CAD build for the part. Positions are in the model's coordinates, mm. Coordinates: 2 decimals unless noted, no trailing zeros. Loops run counter-clockwise (first coordinate to the right, second up) from the corner with the lowest first, then second, coordinate; pieces in that order, holes last. Notation, with made-up numbers: (82.25, -34.75) -> (111.25, -34.75) arc R18 ccw to (111.25, -8.75) -> close; hole circle Ø9 at (20.25, 1.25). An arc over 180 degrees is marked (long way). Return JSON: item names as keys, results as strings. Group by question number.
(1) Saw through at B-B on z = 2.4. Give the number of separate pieces and of enclosed holes in the cut face, then the cut area to 3 significant figures.
(2) Mould opens along Y. For faces 1 (the face through (341, 24, 3.175)), 2 (the face through (88.79, 91.45, 1.57)) say: pulls with the +Y half, pulls with the -Y half, needs draft (parallel to the pull), parting line crosses it, or undercut.
(3) Saw through at A-A on x = 53.34. Write the cut outline in (y, z) (1 decimal), then the cut area to 3 significant figures.
(4) Flat gauge pin, fed straight in: pin 1 Ø1.5 at (x, z) = (300.5, 1.5) entering from +Y. Where does the tip first touch, or does it go through?
(5) Probe L1, parallel to X at y = -10, z = 0.2; L2, parallel to Y at x = 595, z = 2.45; L3, parallel to Y at x = 549, z = 2.2. List the from-to ranges inside material, lowest first.
Autodesk Inventor part; units mm, degrees
ref_plane "YZ Plane" through (0, 0, 0) normal (1, 0, 0) x (0, 1, 0)
ref_plane "XZ Plane" through (0, 0, 0) normal (0, 1, 0) x (-1, 0, 0)
ref_plane "XY Plane" through (0, 0, 0) normal (0, 0, 1) x (1, 0, 0)
sketch "Sketch1" plane through (0, 0, 0) normal (0, 0, 1) x (1, 0, 0)
  line L0 (342.9, 44.45) -> (342.9, 717.1861) construction
  line L1 (-606.2082, 101.6) -> (1077.8216, 101.6) construction
  line L2 (-65.7713, 44.45) -> (606.7605, 44.45) construction
  line L3 (-222.4708, -127) -> (709.547, -127) construction
  arc A0 (684.6761, -149.4566) -> (3.1862, 101.5935) centre (-0.5715, -959.104) ccw
  arc A1 (680.5362, -179.3945) -> (3.1635, 76.1934) centre (-0.5715, -959.104) ccw
  line L4 (0, 98.4185) -> (0, 79.3684)
  arc A2 (3.1862, 101.5935) -> (0, 98.4185) centre (3.175, 98.4185) ccw
  arc A3 (0, 79.3684) -> (3.1635, 76.1934) centre (3.175, 79.3684) ccw
  line L5 (685.8, 390.8172) -> (685.8, -177.0033) construction
  line L6 (657.225, 88.3294) -> (657.225, -181.9974) construction
  line L7 (685.8, -177.0033) -> (685.8, -151.8801)
  arc A4 (685.8, -151.8801) -> (684.6761, -149.4566) centre (682.625, -151.8801) ccw
  arc A5 (680.5362, -179.3945) -> (685.8, -177.0033) centre (682.625, -177.0033) ccw
  point P0 (0, 0)
  point P1 (0, 101.6)
  point P2 (850.5097, -369.5996)
  point P3 (0, 76.2)
  point P4 (685.8, -184.0241)
  point P5 (657.225, -127)
  point P6 (685.8, -150.4091)
  dimension "d2" = 342.9
  dimension "d3" = 101.6
  dimension "d4" = 44.45
  dimension "d6" = 127
  dimension "d7" = 25.4
  dimension "d9" = 3.175
  dimension "d20" = 685.8
  dimension "d21" = 657.225
  dimension "d22" = 3.175
extrude "Extrusion1" add sketch "Sketch1" along normal blind 3.175
sketch "Sketch2" plane through (0, 0, 0) normal (0, 0, -1) x (-1, 0, 0)
  line L0 (0, 79.3684) -> (0, 98.4185)
  circle A0 centre (-12.7, 88.9) radius 2.0701
  circle A1 centre (-673.1, -165.1) radius 2.0701
  point P0 (0, 0)
  dimension "d12" = 4.1402
  dimension "d13" = 12.7
  dimension "d14" = 88.9
  dimension "d15" = 4.1402
  dimension "d17" = 165.1
  dimension "d23" = 673.1
extrude "Extrusion2" cut sketch "Sketch2" against normal blind 25.4
sketch "Sketch3" plane through (0, 0, 0) normal (0, 0, -1) x (-1, 0, 0)
  arc A0 (-3.1862, 101.5935) -> (-684.6761, -149.4566) centre (0.5715, -959.104) ccw
  arc A1 (-3.1635, 76.1934) -> (-680.5362, -179.3945) centre (0.5715, -959.104) ccw
  line L0 (0, 79.3684) -> (0, 98.4185)
  circle A2 centre (-36.0033, 88.2616) radius 6.35
  line L1 (-36.0033, 88.2616) -> (0.5715, -959.104) construction
  line L2 (0.5715, -959.104) -> (0.5715, -266.0692) construction
  line L3 (0.5715, -959.104) -> (-683.9382, -148.8325) construction
  circle A3 centre (-53.34, 87.5124) radius 6.35
  circle A4 centre (-70.662, 86.4763) radius 6.35
  circle A5 centre (-87.9644, 85.1535) radius 6.35
  circle A6 centre (-105.2426, 83.5444) radius 6.35
  circle A7 centre (-122.4917, 81.6495) radius 6.35
  circle A8 centre (-139.7071, 79.4692) radius 6.35
  circle A9 centre (-156.8841, 77.0042) radius 6.35
  circle A10 centre (-174.0178, 74.2551) radius 6.35
  circle A11 centre (-191.1037, 71.2226) radius 6.35
  circle A12 centre (-208.1371, 67.9077) radius 6.35
  circle A13 centre (-225.1132, 64.3113) radius 6.35
  circle A14 centre (-242.0275, 60.4342) radius 6.35
  circle A15 centre (-258.8752, 56.2776) radius 6.35
  circle A16 centre (-275.6518, 51.8426) radius 6.35
  circle A17 centre (-292.3527, 47.1305) radius 6.35
  circle A18 centre (-308.9733, 42.1424) radius 6.35
  circle A19 centre (-325.509, 36.8799) radius 6.35
  circle A20 centre (-341.9553, 31.3443) radius 6.35
  circle A21 centre (-358.3077, 25.5371) radius 6.35
  circle A22 centre (-374.5617, 19.46) radius 6.35
  circle A23 centre (-390.7128, 13.1146) radius 6.35
  circle A24 centre (-406.7567, 6.5026) radius 6.35
  circle A25 centre (-422.6889, -0.3741) radius 6.35
  circle A26 centre (-438.505, -7.5136) radius 6.35
  circle A27 centre (-454.2008, -14.9141) radius 6.35
  circle A28 centre (-469.7718, -22.5734) radius 6.35
  circle A29 centre (-485.214, -30.4895) radius 6.35
  circle A30 centre (-500.5229, -38.6602) radius 6.35
  circle A31 centre (-515.6944, -47.0832) radius 6.35
  circle A32 centre (-530.7245, -55.7563) radius 6.35
  circle A33 centre (-545.6088, -64.6771) radius 6.35
  circle A34 centre (-560.3434, -73.8431) radius 6.35
  circle A35 centre (-574.9242, -83.2518) radius 6.35
  circle A36 centre (-589.3472, -92.9006) radius 6.35
  circle A37 centre (-603.6085, -102.787) radius 6.35
  circle A38 centre (-617.7042, -112.908) radius 6.35
  circle A39 centre (-631.6303, -123.2611) radius 6.35
  circle A40 centre (-645.3831, -133.8434) radius 6.35
  circle A41 centre (-658.9588, -144.6519) radius 6.35
  point P0 (0, 0)
  dimension "d24" = 12.7
  dimension "d25" = 1048.004
  dimension "d26" = 2
  dimension "d27" = 40.191
  dimension "d30" = 37
extrude "Extrusion3" cut sketch "Sketch3" against normal blind 25.4
properties part number "Ramp" material "Aluminum 6061"
Geometry results:
{
 "1": {"separate pieces": "1", "enclosed holes": "42", "area": "13,900 mm²"},
 "2": {"face 1": "needs draft", "face 2": "undercut"},
 "3": {"outline": "(74.8, 0) -> (81.2, 0) -> (81.2, 3.2) -> (74.8, 3.2) -> close; (93.9, 0) -> (100.2, 0) -> (100.2, 3.2) -> (93.9, 3.2) -> close", "area": "40.4 mm²"},
 "4": {"pin 1": "y = 58.2"},
 "5": {"L1": "413.02 to 432.66, 444.35 to 450.18, 458.22 to 473.03", "L2": "-112.26 to -95.79, -90.01 to -81.39", "L3": "-81.71 to -70.05, -59.31 to -51.88"}
}
